Autodesk Inventor part; units mm, degrees
ref_plane "Work Plane1" through (0, 0, 0) normal (1, 0, 0) x (0, 0, -1)
ref_plane "YZ Plane" through (0, 0, 0) normal (1, 0, 0) x (0, 1, 0)
ref_plane "XZ Plane" through (0, 0, 0) normal (0, 1, 0) x (-1, 0, 0)
sketch "Sketch1" plane through (0, 0, 0) normal (0, 1, 0) x (-1, 0, 0)
  circle A0 centre (0, 0) radius 13.25
  circle A1 centre (0, 0) radius 25.25
  circle A2 centre (0, 0) radius 28.25
  dimension "d0" = 26.5
  dimension "d1" = 12
  dimension "d2" = 3
extrude "Extrusion1" add sketch "Sketch1" along normal blind 16 contours A2
extrude "Extrusion2" add sketch "Sketch1" along normal blind 10.5 contours A1
sketch "Sketch2" plane through (0, 10.5, 0) normal (0, 1, 0) x (1, 0, 0)
  line L0 (0, -8) -> (20.25, -8)
  line L1 (20.25, -8) -> (20.25, 8)
  line L2 (20.25, 8) -> (0, 8)
  line L3 (0, 8) -> (0, -8)
  circle A0 centre (0, 0) radius 13.25
  line L4 (0, -8) -> (-20.25, -8)
  line L5 (-20.25, -8) -> (-20.25, 8)
  line L6 (-20.25, 8) -> (0, 8)
  point P0 (10.5623, 8)
  point P1 (10.5623, -8)
  point P2 (-10.5623, -8)
  point P3 (-10.5623, 8)
  dimension "d7" = 20.25
  dimension "d8" = 0
  dimension "d9" = 16
extrude "Extrusion3" cut sketch "Sketch2" against normal blind 10.5 contours A0 L2 L1 L0 | L4 L5 L6 A0
sketch "Sketch3" plane through (-20.25, 10.5, 8) normal (1, 0, 0) x (0, 0, -1)
  circle A0 centre (8, -5.25) radius 2.49
  line L0 (0, 0) -> (16, 0)
  line L1 (0, 0) -> (0, -10.5)
  point P0 (8, -10.5)
  point P1 (8, 0)
  point P2 (0, -5.25)
  dimension "d12" = 4.98
  dimension "d13" = 0
  dimension "d14" = 0
extrude "Extrusion4" add sketch "Sketch3" along normal blind 5.25
chamfer "Chamfer1" distance 0.5 angle 45 1 edges at (-15, 5.25, 2.49)
ref_plane "Work Plane1" through (0, 0, 0) normal (1, 0, 0) x (0, 0, -1)
mirror "Mirror1" about plane through (0, 0, 0) normal (1, 0, 0) of "Extrusion4", "Chamfer1"
sketch "Sketch4" plane through (0, 0, 0) normal (0, -1, 0) x (1, 0, 0)
  circle A0 centre (0, 0) radius 28.25
  line L0 (20.25, -8) -> (10.5623, -8)
  line L1 (-20.25, 8) -> (-10.5623, 8)
  line L2 (20.25, -8) -> (-20.25, -8)
  line L3 (-20.25, -8) -> (-20.25, 8)
  line L4 (-20.25, 8) -> (20.25, 8)
  line L5 (20.25, 8) -> (20.25, -8)
  circle A1 centre (0, 0) radius 13.25
  point P0 (10.5623, 8)
  point P1 (-10.5623, -8)
extrude "Extrusion5" add sketch "Sketch4" along normal blind 5
sketch "Sketch5" plane through (0, -5, 0) normal (0, -1, 0) x (1, 0, 0)
  circle A0 centre (0, 0) radius 13.25
  circle A1 centre (0, 0) radius 18.25
  circle A2 centre (0, 0) radius 44.25
  dimension "d22" = 5
  dimension "d23" = 26
extrude "Extrusion6" add sketch "Sketch5" along normal blind 40 contours A1
extrude "Extrusion7" add sketch "Sketch5" along normal blind 7 contours A2
sketch "Sketch6" plane through (0, -12, 0) normal (0, -1, 0) x (1, 0, 0)
  circle A0 centre (0, 38.325) radius 3.15
  point P0 (0, 0)
  dimension "d28" = 6.3
  dimension "d29" = 38.325
extrude "Extrusion8" add sketch "Sketch6" along normal blind 7
sketch "Sketch7" plane through (0, -12, 0) normal (0, -1, 0) x (1, 0, 0)
  circle A0 centre (0, 0) radius 28.25
  line L0 (0, -28.25) -> (0, -44.25)
  circle A1 centre (0, 0) radius 44.25
  circle A2 centre (0, -36.25) radius 2
  circle A3 centre (31.3934, 18.125) radius 2
  circle A4 centre (-31.3934, 18.125) radius 2
  dimension "d32" = 4
  dimension "d35" = 360
extrude "Extrusion9" cut sketch "Sketch7" against normal blind 7 contours A2 L0 | L0 A2 | A3 | A4
chamfer "Chamfer2" distance 1.5 angle 45 3 edges at (29.3934, -5, 18.125) (-33.3934, -5, 18.125) (-2, -5, -36.25)
properties part number "birdhouse_holder_v1"
Input: part model. Units: mm. Frame: model coordinates. A direction names the side the tool comes from. Give positions to 0.01 mm unless a question says otherwise; leave off trailing zeros. Order: outer loops, then holes, each group sorted by start corner. A loop starts at its lowest first (then second) coordinate and runs counter-clockwise, first axis right, second up. Notation, with made-up numbers: M 36.25,58 L 64.25,58 A34 ccw 64.25,94 Z; hole C -9,-12.5 d1. An arc over 180 degrees is marked long. Return JSON: item names as keys, results as strings.
Item 1: First-contact query: P1, Ø4, axis at x = -18, z = 2, coming from the +Y side; P2, Ø4, axis at x = -24.5, y = 2.5, coming from the +Z side; P3, Ø5, axis at x = -15, y = 4, coming from the -Z side; P4, Ø1.5, axis at y = -4, z = 34, coming from the +X side. Flat tips, straight axial feed; report the tip coordinate or a pass-through.
Solutions:
{"P1": "y = 7.74", "P2": "z = 17.08", "P3": "z = -25.33", "P4": "through"}
Item 2: Pull-direction query (Z, two-part tool) for faces 4 (the flat face through (21, 16, -15)), 5 (the flat face through (-15, 5, 0)); classes: +Z half, -Z half, draft (parallel to the pull), parting line (faces both ways), or undercut.
Solutions:
{"face 4": "draft", "face 5": "undercut"}
Item 3: Cut plane C-C (z = -36.25). Return loops of the section in (x, y), then the cut area to 3 significant figures.
Solutions:
{"outline": "M -25.38,-12 L -2,-12 L -2,-6.5 L -3.5,-5 L -25.38,-5 Z; M 2,-12 L 25.38,-12 L 25.38,-5 L 3.5,-5 L 2,-6.5 Z", "area": "325 mm^2"}
Item 4: Cut plane D-D (y = -14). Return loops of the section in (x, z) (3 decimals).
Solutions:
{"outline": "C 0,0 d36.5; C 0,38.325 d6.3; hole C 0,0 d26.5"}
Item 5: Cut plane A-A (x = 0). State how many separate pieces and enclosed holes the cut face has, then the cut area to 3 significant figures.
Solutions:
{"separate pieces": "3", "enclosed holes": "0", "area": "1,280 mm^2"}
Item 6: Ray query, probe 1 along Y at (x, z) = (-36.5, 12.5); probe 2 along Z at (x, y) = (0, 14); probe 3 along X at (y, z) = (-8.3, -36.25). Return the intervals inside material, ascending.
Solutions:
{"probe 1": "-12 to -5", "probe 2": "-28.25 to -25.25, 25.25 to 28.25", "probe 3": "-25.38 to -2, 2 to 25.38"}
Item 7: Cut plane B-B (y = 5.25). Return loops of the section in (x, z), then the cut area to 3 significant figures.
Solutions:
{"outline": "C 0,0 d56.5; hole M -20.25,-8 L -10.56,-8 A13.25 ccw 10.56,-8 L 20.25,-8 L 20.25,-2.49 L 15.5,-2.49 L 15,-1.99 L 15,1.99 L 15.5,2.49 L 20.25,2.49 L 20.25,8 L 10.56,8 A13.25 ccw -10.56,8 L -20.25,8 L -20.25,2.49 L -15.5,2.49 L -15,1.99 L -15,-1.99 L -15.5,-2.49 L -20.25,-2.49 Z", "area": "1,760 mm^2"}
Item 8: Access query for faces 1 (the cylindrical face through (17.91, 2.82, 0.54)), 2 (the cylindrical face through (-0.68, -15.45, 41.4)), 3 (the flat face through (-11, 10.5, -11)). Directions: +Z, -Z, +X, -X, +Y, -Y. A direction counts if a zero-diameter tool reaches every point of the face in a straight line with its end or side. Return the directions, or none.
Solutions:
{"face 1": "none", "face 2": "-Y", "face 3": "+Y"}
